Source: CAD feature listing. Evaluate the final solid. Frame: model axes, mm. A direction names the side the tool comes from. Round coordinates to 2 decimals unless told otherwise and drop trailing zeros. Order: outer loops, then holes, each group sorted by start corner. A loop starts at its lowest first (then second) coordinate and runs counter-clockwise, first axis right, second up. Notation, with made-up numbers: M 47.5,58.25 L 70.5,58.25 A12 ccw 70.5,73.25 Z; hole C 27.25,-6.5 d5. An arc over 180 degrees is marked long. Use one line per item in the form item = value. Start each with the question number.
Q1. Reachability of faces 1 (the flat face through (0, 16.7, -95)), 2 (the flat face through (0, 16.7, 410)), 3 (the flat face through (20.1, 1.6, 284)), 4 (the cylindrical face through (-1.08, -4.88, -127.18)) from +Z, -Z, +X, -X, +Y, -Y: full face, straight path, thin tool, end or side. Return the list, or none.
Q2. Material intervals for probe 1 along Y at (x, z) = (0, 410); probe 2 along Y at (x, z) = (1.5, -38.5); probe 3 along Z at (x, y) = (-13, 18), sorted ascending.
Q3. Section A-A (z = -9.5). Return the cut outline in (x, y).
Q4. Section D-D (z = 184.5). Return the cut outline in (x, y).
Q5. Pull-direction query (Y, two-part tool) for faces 5 (the flat face through (-22.34, 3.82, 234)), 6 (the flat face through (0, 0, 394)), 7 (the cylindrical face through (-10.752, -16.864, 362.585)); classes: pulls with the +Y half, pulls with the -Y half, needs draft (parallel to the pull), parting line crosses it, or undercut.
Q6. Contact query for flat-ended pins moving along their axis: pin 1 (9 mm diameter, centred on x = 0, y = 0, fed in from +Z); pin 2 (2 mm diameter, centred on x = 7, z = 138, fed in from +Y); pin 3 (3 mm diameter, centred on x = -17, z = 322.5, fed in from +Y). Output: stop coordinate, or through.
Q7. Section B-B (x = -11.5). Return the cut outline in (y, z), plus the area to 3 significant figures.
Q8. Section C-C (y = -14). Return the cut outline in (x, z), plus the area to 3 significant figures.
from build123d import *

# Parameters (mm, degrees)
SKETCH1_R                  = 25
BOSS_EXTRUDE1_DEPTH        = 234
SKETCH2_R                  = 22.5
BOSS_EXTRUDE2_DEPTH        = 40
SKETCH3_R                  = 20
BOSS_EXTRUDE3_DEPTH        = 110
BOSS_EXTRUDE4_START        = 50
SKETCH4_R                  = 22.5
BOSS_EXTRUDE4_DEPTH        = 50
BOSS_EXTRUDE5_START        = 155
SKETCH5_R                  = 20
BOSS_EXTRUDE5_DEPTH        = 155
CUT_EXTRUDE1_DEPTH         = 3.3
SKETCH7_R                  = 5
CUT_EXTRUDE2_DEPTH         = 45
CUT_EXTRUDE3_DEPTH         = 3.3
F_10_0MM_DOWEL_HOLE1_D     = 10
F_10_0MM_DOWEL_HOLE1_DEPTH = 45
F_10_0MM_DOWEL_HOLE1_TIP   = 3.004303095


with BuildPart() as part:
    # Sketch1 → Boss-Extrude1 (new body)
    with BuildSketch(Plane.XY):
        Circle(SKETCH1_R)
    extrude(amount=BOSS_EXTRUDE1_DEPTH)

    # Sketch2 → Boss-Extrude2 (add)
    with BuildSketch(Plane(origin=(0, 0, 0), x_dir=(-1, 0, 0), z_dir=(0, 0, -1))):
        Circle(SKETCH2_R)
    extrude(amount=BOSS_EXTRUDE2_DEPTH)

    # Sketch3 → Boss-Extrude3 (add)
    with BuildSketch(Plane(origin=(0, 0, -40), x_dir=(-1, 0, 0), z_dir=(0, 0, -1))):
        Circle(SKETCH3_R)
    extrude(amount=BOSS_EXTRUDE3_DEPTH)

    # Sketch4 → Boss-Extrude4 (add)
    with BuildSketch(Plane.XY.offset(234).offset(BOSS_EXTRUDE4_START)):
        with Locations(Location((0, 0, 0), (0, 0, 180))):
            Circle(SKETCH4_R)
    extrude(amount=-BOSS_EXTRUDE4_DEPTH)

    # Sketch5 → Boss-Extrude5 (add)
    with BuildSketch(Plane.XY.offset(284).offset(BOSS_EXTRUDE5_START)):
        with Locations(Location((0, 0, 0), (0, 0, 180))):
            Circle(SKETCH5_R)
    extrude(amount=-BOSS_EXTRUDE5_DEPTH)

    # Sketch6 → Cut-Extrude1 (cut)
    with BuildSketch(Plane(origin=(0, 20, 0), x_dir=(1, 0, 0), z_dir=(0, 1, 0))):
        with BuildLine():
            Line((-6, -439), (-6, -388))
            ThreePointArc((-6, -388), (0, -382), (6, -388))
            Line((6, -388), (6, -439))
            ThreePointArc((6, -439), (0, -445), (-6, -439))
        make_face()
    extrude(amount=-CUT_EXTRUDE1_DEPTH, mode=Mode.SUBTRACT)

    # Sketch7 → Cut-Extrude2 (cut)
    with BuildSketch(Plane.XY.offset(439)):
        Circle(SKETCH7_R)
    extrude(amount=-CUT_EXTRUDE2_DEPTH, mode=Mode.SUBTRACT)

    # Sketch8 → Cut-Extrude3 (cut)
    with BuildSketch(Plane(origin=(0, 20, 0), x_dir=(1, 0, 0), z_dir=(0, 1, 0))):
        with BuildLine():
            Line((6, 138), (6, 50))
            ThreePointArc((6, 50), (0, 44), (-6, 50))
            Line((-6, 50), (-6, 138))
            ThreePointArc((-6, 138), (0, 144), (6, 138))
        make_face()
    extrude(amount=-CUT_EXTRUDE3_DEPTH, mode=Mode.SUBTRACT)

    # Ø10.0mm Dowel Hole1
    with Locations(Plane(origin=(0, 0, -150), x_dir=(-1, 0, 0), z_dir=(0, 0, -1))):
        with Locations((0, 0)):
            Hole(F_10_0MM_DOWEL_HOLE1_D / 2, depth=F_10_0MM_DOWEL_HOLE1_DEPTH)
            with Locations((0, 0, -(F_10_0MM_DOWEL_HOLE1_DEPTH + F_10_0MM_DOWEL_HOLE1_TIP / 2))):  # 118° drill point
                Cone(0, F_10_0MM_DOWEL_HOLE1_D / 2, F_10_0MM_DOWEL_HOLE1_TIP, mode=Mode.SUBTRACT)


solid = part.part
Results list:
q1.face_1 = +Y
q1.face_2 = +Z, +Y
q1.face_3 = +Z
q1.face_4 = -Z
q2.probe_1 = -20 to -5, 5 to 16.7
q2.probe_2 = -22.45 to 22.45
q2.probe_3 = -40 to 284
q3.outline = C 0,0 d45
q4.outline = C 0,0 d50
q5.face_5 = needs draft
q5.face_6 = undercut
q5.face_7 = parting line crosses it
q6.pin_1 = 394
q6.pin_2 = 24.27
q6.pin_3 = 12.64
q7.outline = M -22.2,0 L -19.34,0 L -19.34,-40 L -16.36,-40 L -16.36,-150 L 16.36,-150 L 16.36,-40 L 19.34,-40 L 19.34,0 L 22.2,0 L 22.2,234 L 19.34,234 L 19.34,284 L 16.36,284 L 16.36,439 L -16.36,439 L -16.36,284 L -19.34,284 L -19.34,234 L -22.2,234 Z
q7.area = 22,500 mm2
q8.outline = M -20.71,0 L -17.61,0 L -17.61,-40 L -14.28,-40 L -14.28,-150 L 14.28,-150 L 14.28,-40 L 17.61,-40 L 17.61,0 L 20.71,0 L 20.71,234 L 17.61,234 L 17.61,284 L 14.28,284 L 14.28,439 L -14.28,439 L -14.28,284 L -17.61,284 L -17.61,234 L -20.71,234 Z
q8.area = 20,400 mm2
